from build123d import *

# Parameters (mm, degrees)
F0_W     = 12.7
F0_H     = 132.08
F1_DEPTH = 3.175
F3_DEPTH = 25.4
F4_DEPTH = 25.4


# Not quite as in the source:
# - a feature names something its author has since deleted; it is built from what else it names


with BuildPart() as f1:
    # F0 (on Top) → F1 (new body)
    with BuildSketch(Plane.XY):
        Polygon((28.5549264625, 56.9072367892), (-98.4450735375, 56.9072367892), (-98.4450735375, 34.0472367892), (-41.2950735375, 34.0472367892), (-28.5950735375, 34.0472367892), (28.5549264625, 34.0472367892), align=None)
        with Locations((-34.9450735375, -31.9927632108)):
            Rectangle(F0_W, F0_H)
        Polygon((-41.2950735375, -98.0327632108), (-98.4450735375, -98.0327632108), (-98.4450735375, -120.8927632108), (28.5549264625, -120.8927632108), (28.5549264625, -98.0327632108), (-28.5950735375, -98.0327632108), align=None)
    extrude(amount=F1_DEPTH)

    # F2 (on face) → F3 (cut)
    with BuildSketch(Plane.XY.offset(3.175)):
        Polygon((28.5549264625, 45.4772367892), (9.7966708748, 45.4772367892), (28.5549264625, 35.3785827756), align=None)
        Polygon((-98.4450735375, 35.3785827756), (-79.6868179499, 45.4772367892), (-98.4450735375, 45.4772367892), align=None)
    extrude(amount=-F3_DEPTH, mode=Mode.SUBTRACT)

    # F2 (on face) → F4 (cut)
    with BuildSketch(Plane.XY.offset(3.175)):
        Polygon((28.5549264625, 55.5758908027), (9.7966708748, 45.4772367892), (28.5549264625, 45.4772367892), align=None)
        Polygon((-98.4450735375, 45.4772367892), (-79.6868179499, 45.4772367892), (-98.4450735375, 55.5758908027), align=None)
    extrude(amount=-F4_DEPTH, mode=Mode.SUBTRACT)


solid = f1.part
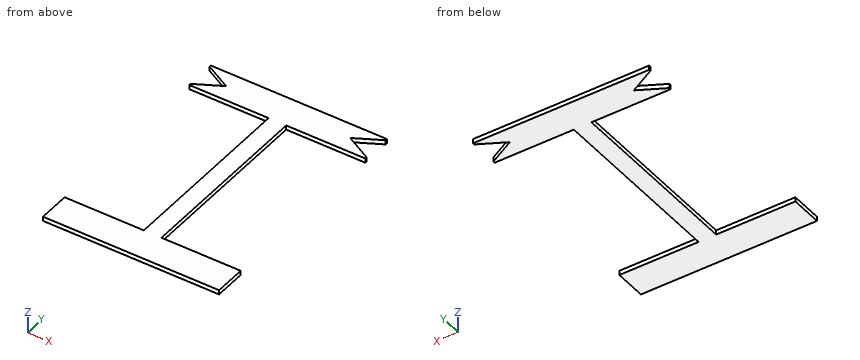
Geometry: final body of the model. Coordinates: model frame, mm. Coordinates: 2 decimals unless noted, no trailing zeros. Loops run counter-clockwise (first coordinate to the right, second up) from the corner with the lowest first, then second, coordinate; pieces in that order, holes last. Notation, with made-up numbers: M 63.5,-4 L 111.5,-4 A26 ccw 111.5,11 Z; hole C 63,19 d10. An arc over 180 degrees is marked long. One line per item, written item: value. Start each with the question number.
1) Cut plane C-C (x = -85). Return loops of the section in (y, z) (3 decimals), then the cut area to 3 significant figures.
2) Cut plane B-B (z = 1). Return loops of the section in (x, y), then the cut area to 4 significant figures.
3) Material intervals for L1, parallel to Y at x = -64, z = 3; L2, parallel to Y at x = -82.5, z = 0.1; L3, parallel to Y at x = 22, z = 3, sorted ascending. Write a range as from..to.
4) Cut plane D-D (y = 28). Return loops of the section in (x, z) (3 decimals), then the cut area to 3 significant figures.
5) Pin query (flat end, axial travel): P1, Ø1, axis at y = -61, z = 1.5, coming from the +X side; P2, Ø1.5, axis at y = 29, z = 1, coming from the -X side. Return the tip coordinate at first contact, or that it passes through.
6) Cut plane A-A (x = -69.5). Return loops of the section in (y, z) (3 decimals).
Evaluation:
1. outline: M -120.893,0 L -98.033,0 L -98.033,3.175 L -120.893,3.175 Z; M 34.047,0 L 42.617,0 L 42.617,3.175 L 34.047,3.175 Z; M 48.338,0 L 56.907,0 L 56.907,3.175 L 48.338,3.175 Z
1. area: 127 mm^2
2. outline: M -98.45,-120.89 L 28.55,-120.89 L 28.55,-98.03 L -28.6,-98.03 L -28.6,34.05 L 28.55,34.05 L 28.55,35.38 L 9.8,45.48 L 28.55,55.58 L 28.55,56.91 L -98.45,56.91 L -98.45,55.58 L -79.69,45.48 L -98.45,35.38 L -98.45,34.05 L -41.3,34.05 L -41.3,-98.03 L -98.45,-98.03 Z
2. area: 7,105 mm^2
3. L1: -120.89..-98.03, 34.05..56.91
3. L2: -120.89..-98.03, 34.05..43.96, 46.99..56.91
3. L3: -120.89..-98.03, 34.05..38.91, 52.05..56.91
4. outline: M -41.295,0 L -28.595,0 L -28.595,3.175 L -41.295,3.175 Z
4. area: 40.3 mm^2
5. P1: x = -28.6
5. P2: x = -41.3
6. outline: M -120.893,0 L -98.033,0 L -98.033,3.175 L -120.893,3.175 Z; M 34.047,0 L 56.907,0 L 56.907,3.175 L 34.047,3.175 Z
